Check sheet for the modelled part. Datum: model origin and axes. Units: mm. A direction names the side the tool comes from. Give positions to 0.01 mm unless a question says otherwise; leave off trailing zeros. Write each loop counter-clockwise with the first axis right and the second up, starting at its lowest first coordinate (ties: lowest second). Pieces come first, ordered by that corner, then holes. Notation, with made-up numbers: M 52,43.5 L 96,43.5 A19 cw 96,78.5 Z; hole C 18,8.5 d6. An arc over 180 degrees is marked long. Write each question's results on one line, items separated by ' | '. Start each with the question number.
from build123d import *

# Parameters (mm, degrees)
F0_R     = 24
F0_R_2   = 15
F1_DEPTH = 20
F2_R     = 24
F3_DEPTH = 10
F5_D     = 4.2
F6_D     = 17.5


with BuildPart() as f1:
    # F0 (on Front) → F1 (new body)
    with BuildSketch(Plane.XZ):
        Circle(F0_R)
        Circle(F0_R_2, mode=Mode.SUBTRACT)
    extrude(amount=F1_DEPTH)

    # F2 (on face) → F3 (join)
    with BuildSketch(Plane.XZ.offset(20)):
        Circle(F2_R)
    extrude(amount=F3_DEPTH)

    # F5 (through all)
    with Locations(Plane(origin=(0, 0, 0), x_dir=(-1, 0, 0), z_dir=(0, 1, 0))):
        with Locations((0, 19), (16.4544826719, 9.5), (16.4544826719, -9.5), (0, -19), (-16.4544826719, -9.5), (-16.4544826719, 9.5)):
            Hole(F5_D / 2)

    # F6 (through all)
    with Locations(Plane(origin=(0, 0, 0), x_dir=(-1, 0, 0), z_dir=(0, 1, 0))):
        with Locations((0, 0)):
            Hole(F6_D / 2)


solid = f1.part
Q1. Depth check by flat-ended pin: pin 1 Ø16 at (x, z) = (0, 0) entering from -Y; pin 2 Ø8 at (y, z) = (-25.5, 12) entering from -X; pin 3 Ø10 at (y, z) = (-18, 16) entering from -X; pin 4 Ø24 at (x, z) = (0, 0) entering from +Y. Enter the tip coordinate at first touch or a pass-through.
Q2. Release check for a two-part mould opening along Z. For faces 3 (the face through (-14.985, -9.86, 0.66)), 4 (the face through (-23.977, -14.79, 1.055)), 5 (the face through (16, 0, 0)) record: pulls with the +Z half, pulls with the -Z half, needs draft (parallel to the pull), parting line crosses it, or undercut.
Q3. Section check A-A on x = 0. Record the boundary of the cut face in (y, z).
Q4. Scan lines: L1, parallel to Z at x = 0, y = -12.5; L2, parallel to Z at x = -17.5, y = -22; L3, parallel to Z at x = 17, y = -27.5. Record each from-to range of solid material in increasing order.
Q5. Section check C-C on z = -10.5. Record the boundary of the cut face in (x, y), plus the area to 3 significant figures.
Q6. Section check D-D on x = 5.5. Record the boundary of the cut face in (y, z), plus the area to 3 significant figures.
Q7. Section check B-B on y = -9.5. Record the boundary of the cut face in (x, z).
Q8. Tool access check on faces 1 (the face through (6.5, -20, -6.5)), 2 (the face through (-6.944, -25.07, -5.324)). Record the directions out of +Z, -Z, +X, -X, +Y, -Y that give a thin tool (end or side, any length) a straight path to the whole face; none if there is none.
Check result:
1) pin 1: through | pin 2: x = -22.63 | pin 3: x = -21.33 | pin 4: y = -20
2) face 3: undercut | face 4: parting line crosses it | face 5: needs draft
3) outline: M -30,-24 L 0,-24 L 0,-21.1 L -30,-21.1 Z; M -30,-16.9 L 0,-16.9 L 0,-15 L -20,-15 L -20,-8.75 L -30,-8.75 Z; M -30,8.75 L -20,8.75 L -20,15 L 0,15 L 0,16.9 L -30,16.9 Z; M -30,21.1 L 0,21.1 L 0,24 L -30,24 Z
4) L1: -24 to -21.1, -16.9 to -15, 15 to 16.9, 21.1 to 24 | L2: -16.42 to -11.32, -7.68 to 7.68, 11.32 to 16.42 | L3: -16.94 to -11.53, -7.47 to 7.47, 11.53 to 16.94
5) outline: M -21.58,-30 L -18.3,-30 L -18.3,0 L -21.58,0 Z; M -14.61,-30 L 14.61,-30 L 14.61,0 L 10.71,0 L 10.71,-20 L -10.71,-20 L -10.71,0 L -14.61,0 Z; M 18.3,-30 L 21.58,-30 L 21.58,0 L 18.3,0 Z | area: 645 mm^2
6) outline: M -30,-23.36 L 0,-23.36 L 0,-13.96 L -20,-13.96 L -20,-6.81 L -30,-6.81 Z; M -30,6.81 L -20,6.81 L -20,13.96 L 0,13.96 L 0,23.36 L -30,23.36 Z | area: 707 mm^2
7) outline: C 0,0 d48; hole C -16.45,-9.5 d4.2; hole C -16.45,9.5 d4.2; hole C 0,0 d30; hole C 0,-19 d4.2; hole C 0,19 d4.2; hole C 16.45,-9.5 d4.2; hole C 16.45,9.5 d4.2
8) face 1: +Y | face 2: +Y, -Y
